Verification items for this drawing (mm, ordinates from the low corner). Give positions to 0.01 mm unless a question says otherwise; leave off trailing zeros. Write each loop counter-clockwise with the first axis right and the second up, starting at its lowest first coordinate (ties: lowest second). Pieces come first, ordered by that corner, then holes. Notation, with made-up numbers: (70.25, -7.75) -> (91.25, -7.75) arc R24 cw to (91.25, 7.25) -> close; hole circle Ø9 at (4.25, 87). An arc over 180 degrees is marked (long way). Answer as a JSON object with one key per item and string values.
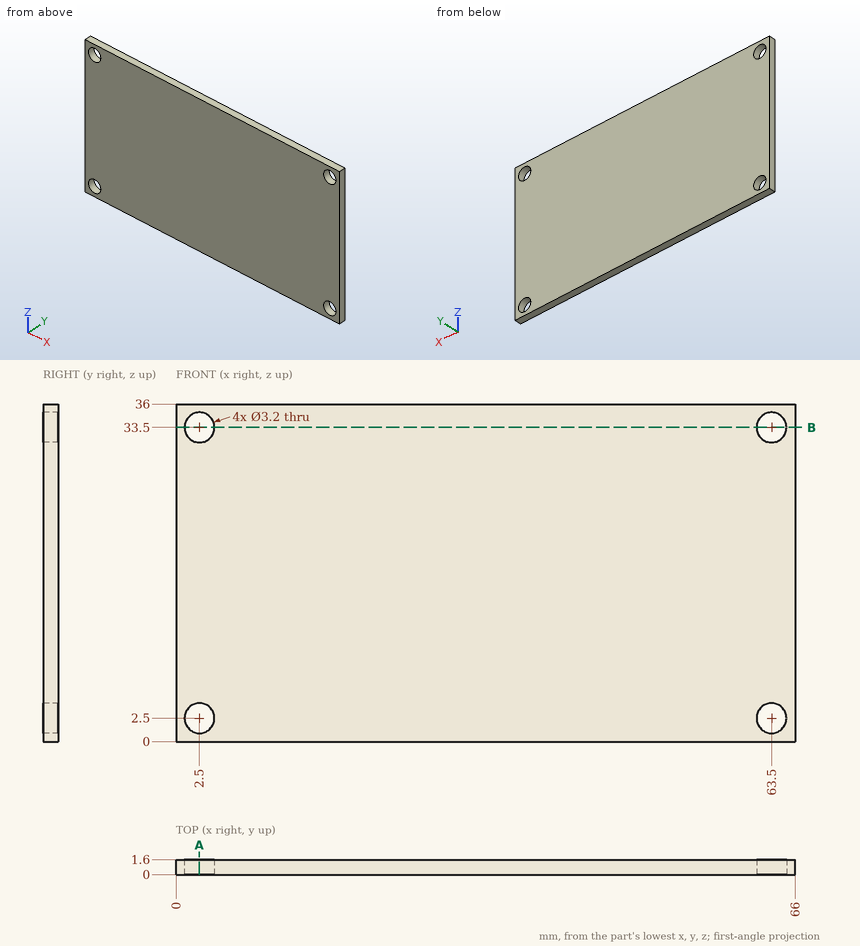
1. Sectioned sample at B-B, the plane z = 33.5. Enter the section's corners in (x, y), plus the area to 3 significant figures.
Determined:
{"outline": "(0, 0) -> (0.9, 0) -> (0.9, 1.6) -> (0, 1.6) -> close; (4.1, 0) -> (61.9, 0) -> (61.9, 1.6) -> (4.1, 1.6) -> close; (65.1, 0) -> (66, 0) -> (66, 1.6) -> (65.1, 1.6) -> close", "area": "95.4 mm^2"}
2. Scan line: L1, parallel to Z at x = 63.5, y = 1.2. Record every from-to range of solid material in increasing order. Write a range as [from, to].
Determined:
{"L1": "[0, 0.9], [4.1, 31.9], [35.1, 36]"}
3. Sectioned sample at A-A, the plane x = 2.5. Enter the section's corners in (y, z), plus the area to 3 significant figures.
Determined:
{"outline": "(0, 0) -> (1.6, 0) -> (1.6, 0.9) -> (0, 0.9) -> close; (0, 4.1) -> (1.6, 4.1) -> (1.6, 31.9) -> (0, 31.9) -> close; (0, 35.1) -> (1.6, 35.1) -> (1.6, 36) -> (0, 36) -> close", "area": "47.4 mm^2"}
